Autodesk Inventor part; units mm, degrees
ref_plane "YZ Plane" through (0, 0, 0) normal (1, 0, 0) x (0, 1, 0)
ref_plane "XZ Plane" through (0, 0, 0) normal (0, 1, 0) x (-1, 0, 0)
ref_plane "XY Plane" through (0, 0, 0) normal (0, 0, 1) x (1, 0, 0)
sketch "Sketch1" plane through (0, 0, 0) normal (0, 1, 0) x (-1, 0, 0)
  line L0 (-2.54, 0) -> (-15.24, 0)
  line L1 (-17.78, -2.54) -> (-17.78, -16.51)
  line L2 (-15.24, -19.05) -> (-2.54, -19.05)
  line L3 (0, -16.51) -> (0, -2.54)
  arc A0 (-2.54, -19.05) -> (0, -16.51) centre (-2.54, -16.51) ccw
  arc A1 (-17.78, -16.51) -> (-15.24, -19.05) centre (-15.24, -16.51) ccw
  arc A2 (0, -2.54) -> (-2.54, 0) centre (-2.54, -2.54) ccw
  arc A3 (-15.24, 0) -> (-17.78, -2.54) centre (-15.24, -2.54) ccw
  circle A4 centre (-2.54, -16.51) radius 1.016
  circle A5 centre (-15.24, -16.51) radius 1.016
  line L4 (0, -2.54) -> (-17.78, -2.54) construction
  circle A6 centre (-1.27, -2.54) radius 0.508
  circle A7 centre (-3.81, -2.54) radius 0.508
  circle A8 centre (-6.35, -2.54) radius 0.508
  circle A9 centre (-8.89, -2.54) radius 0.508
  circle A10 centre (-11.43, -2.54) radius 0.508
  circle A11 centre (-13.97, -2.54) radius 0.508
  circle A12 centre (-16.51, -2.54) radius 0.508
  point P0 (0, 0)
  point P1 (-17.78, -19.05)
  point P2 (-17.78, 0)
  point P3 (0, -19.05)
  dimension "d0" = 17.78
  dimension "d1" = 19.05
  dimension "d2" = 2.54
  dimension "d3" = 2.032
  dimension "d6" = 2.54
  dimension "d11" = 1.27
  dimension "d12" = 1.27
  dimension "d13" = 1.016
  dimension "d16" = 2.54
extrude "Extrusion1" add sketch "Sketch1" along normal blind 1.65
properties part number "BMP280 footprint"
Geometry: final body of the model. Coordinates: model frame, mm. Coordinates: 2 decimals unless noted, no trailing zeros. Loops run counter-clockwise (first coordinate to the right, second up) from the corner with the lowest first, then second, coordinate; pieces in that order, holes last. Notation, with made-up numbers: M -2,54.5 L 30,54.5 A21 ccw 30,61.5 Z; hole C 15.5,-29.5 d3. An arc over 180 degrees is marked long. Put each result on its own line as item: value.
(1) Material intervals for probe 1 along Z at (x, y) = (13.97, 0.8); probe 2 along Z at (x, y) = (2.54, 0.6); probe 3 along X at (y, z) = (0.5, -16), sorted ascending.
Answer sheet:
probe 1: z = -19.05 to -3.05, -2.03 to 0
probe 2: z = -19.05 to -17.53, -15.49 to 0
probe 3: x = 0 to 1.66, 3.42 to 14.36, 16.12 to 17.78
(2) Cut plane A-A on x = 6.35. Return the cut outline in (y, z), then the cut area to 3 significant figures.
Answer sheet:
outline: M 0,-19.05 L 1.65,-19.05 L 1.65,-3.05 L 0,-3.05 Z; M 0,-2.03 L 1.65,-2.03 L 1.65,0 L 0,0 Z
area: 29.8 mm^2
(3) Cut plane B-B on y = 0.5. State how many separate pieces and enclosed holes the cut face has, then the cut area to 3 significant figures.
Answer sheet:
separate pieces: 1
enclosed holes: 9
area: 321 mm^2
(4) Draft query along Z for faces 1 (the face through (9, 1, 0)), 2 (the face through (4.318, 0.813, -2.562)), 3 (the face through (0, 1, -10)). Return one class per face: pulls with the +Z half, pulls with the -Z half, needs draft (parallel to the pull), parting line crosses it, or undercut.
Answer sheet:
face 1: pulls with the +Z half
face 2: undercut
face 3: needs draft
(5) Cut plane C-C on x = 1.27. Return the cut outline in (y, z), then the cut area to 3 significant figures.
Answer sheet:
outline: M 0,-18.71 L 1.65,-18.71 L 1.65,-3.05 L 0,-3.05 Z; M 0,-2.03 L 1.65,-2.03 L 1.65,-0.34 L 0,-0.34 Z
area: 28.6 mm^2
